Geometry: final body of the model. Coordinates: model frame, mm. Face numbers are marked on the shaded views. A direction names the side the tool comes from. Coordinates: 2 decimals unless noted, no trailing zeros. Order: outer loops, then holes, each group sorted by start corner. A loop starts at its lowest first (then second) coordinate and runs counter-clockwise, first axis right, second up. Notation, with made-up numbers: (40, -25) -> (86, -25) arc R24 cw to (86, -3) -> close; hole circle Ø7 at (85.5, 36). An arc over 180 degrees is marked (long way). Use one line per item in the form item = value.
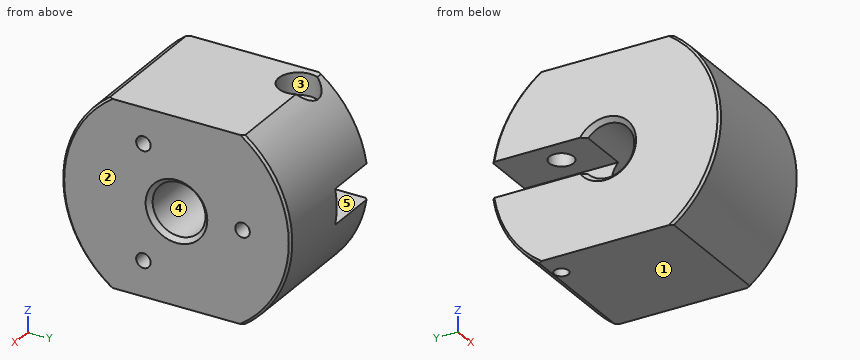
```python
from build123d import *

# Parameters (mm, degrees)
BOSS_EXTRUDE1_DEPTH                     = 30
CUT_EXTRUDE1_DEPTH                      = 12.5
SKETCH3_W                               = 30
SKETCH3_H                               = 6
HOLE1_D                                 = 5.08
HOLE1_DEPTH                             = 8.413530316
HOLE1_TIP                               = 1.466469684
SKETCH6_W                               = 1.621
SKETCH6_H                               = 17
CBORE_FOR_M5_HEX_HEAD_BOLT1_D           = 5.5118
CBORE_FOR_M5_HEX_HEAD_BOLT1_DEPTH       = 17
CBORE_FOR_M5_HEX_HEAD_BOLT1_CBORE_D     = 9
CBORE_FOR_M5_HEX_HEAD_BOLT1_CBORE_DEPTH = 5
CHAMFER1_SIZE                           = 0.5
CHAMFER2_SIZE                           = 1
CHAMFER3_SIZE                           = 0.379
M4_TAPPED_HOLE1_D                       = 3.3
M4_TAPPED_HOLE1_DEPTH                   = 8
M4_TAPPED_HOLE1_TIP                     = 0.991420021


with BuildPart() as part:
    # Sketch1 → Boss-Extrude1 (new body)
    with BuildSketch(Plane(origin=(0, 0, 0), x_dir=(0, 0, -1), z_dir=(1, 0, 0))):
        with BuildLine():
            Line((21, -15.329709717), (21, 15.329709717))
            ThreePointArc((21, 15.329709717), (0, 26), (-21, 15.329709717))
            Line((-21, 15.329709717), (-21, -15.329709717))
            ThreePointArc((-21, -15.329709717), (0, -26), (21, -15.329709717))
        make_face()
    extrude(amount=-BOSS_EXTRUDE1_DEPTH)

    # Sketch2 → Cut-Extrude1 (cut)
    with BuildSketch(Plane.ZY.offset(30)):
        with BuildLine():
            Line((-4, 25.690465157), (-4, 4.472135955))
            ThreePointArc((-4, 4.472135955), (0, 6), (4, 4.472135955))
            Line((4, 4.472135955), (4, 25.690465157))
            ThreePointArc((4, 25.690465157), (0, 26), (-4, 25.690465157))
        make_face()
    extrude(amount=-CUT_EXTRUDE1_DEPTH, mode=Mode.SUBTRACT)

    # Sketch3 → Cut-Revolve1 (revolve, cut)
    with BuildSketch(Plane.XY):
        with Locations((-15, 3)):
            Rectangle(SKETCH3_W, SKETCH3_H)
    revolve(axis=Axis((-30, 0, 0), (1, 0, 0)), mode=Mode.SUBTRACT)

    # Hole1
    with Locations(Plane.ZY.offset(17.5)):
        with Locations((0, 21.27272472)):
            Hole(HOLE1_D / 2, depth=HOLE1_DEPTH)
            with Locations((0, 0, -(HOLE1_DEPTH + HOLE1_TIP / 2))):  # 120° drill point
                Cone(0, HOLE1_D / 2, HOLE1_TIP, mode=Mode.SUBTRACT)

    # Sketch6 → M3 Clearance Hole1 (revolve, cut)
    with BuildSketch(Plane(origin=(-24, 13.5, -4), x_dir=(0, -1, 0), z_dir=(1, 0, 0))):
        with Locations((0.8105, 8.5)):
            Rectangle(SKETCH6_W, SKETCH6_H)
    revolve(axis=Axis((-24, 13.5, 2.35), (0, 0, -1)), mode=Mode.SUBTRACT)

    # CBORE for M5 Hex Head Bolt1
    with Locations(Plane.XY.offset(21)):
        with Locations((-24, 13.5)):
            CounterBoreHole(CBORE_FOR_M5_HEX_HEAD_BOLT1_D / 2, CBORE_FOR_M5_HEX_HEAD_BOLT1_CBORE_D / 2, CBORE_FOR_M5_HEX_HEAD_BOLT1_CBORE_DEPTH, depth=CBORE_FOR_M5_HEX_HEAD_BOLT1_DEPTH)

    # Chamfer1
    chamfer1_edges = [part.edges().sort_by_distance(p)[0] for p in [
        (-30, 22.201659548, -13.530939115),
        (-30, 22.201659548, 13.530939115),
        (-30, -26, 0),
        (0, 26, 0),
        (0, -26, 0),
    ]]
    chamfer(chamfer1_edges, length=CHAMFER1_SIZE)

    # Chamfer2
    chamfer2_edges = [part.edges().sort_by_distance(p)[0] for p in [
        (-30, -6, 0),
        (0, -6, 0),
    ]]
    chamfer(chamfer2_edges, length=CHAMFER2_SIZE)

    # Chamfer3
    chamfer3_edges = [part.edges().sort_by_distance(p)[0] for p in [
        (-24, 15.121, -4),
    ]]
    chamfer(chamfer3_edges, length=CHAMFER3_SIZE)

    # M4 Tapped Hole1
    with Locations(Plane(origin=(0, 0, 0), x_dir=(0, 0, -1), z_dir=(1, 0, 0))):
        with Locations((0, 15), (12.990381057, -7.5), (-12.990381057, -7.5), (0, 0)):
            Hole(M4_TAPPED_HOLE1_D / 2, depth=M4_TAPPED_HOLE1_DEPTH)
            with Locations((0, 0, -(M4_TAPPED_HOLE1_DEPTH + M4_TAPPED_HOLE1_TIP / 2))):  # 118° drill point
                Cone(0, M4_TAPPED_HOLE1_D / 2, M4_TAPPED_HOLE1_TIP, mode=Mode.SUBTRACT)


solid = part.part
```
1) Access query for the marked faces 4 and 5. Directions: +Z, -Z, +X, -X, +Y, -Y. A direction counts if a zero-diameter tool reaches every point of the face in a straight line with its end or side. Return the directions, or none.
Results found:
face_4 = +X, -X
face_5 = -X, +Y
2) Section C-C, the plane x = -24. Output: boundary loops of the cut face in (y, z).
Results found:
outline = (-15.33, -21) -> (11.88, -21) -> (11.88, -4.38) -> (11.5, -4) -> (4.47, -4) arc R6 cw (long way) to (4.47, 4) -> (10.74, 4) -> (10.74, 16) -> (9, 16) -> (9, 21) -> (-15.33, 21) arc R26 ccw to start; (15.12, -21) -> (15.33, -21) arc R26 ccw to (25.69, -4) -> (15.5, -4) -> (15.12, -4.38) -> close; (16.26, 4) -> (25.69, 4) arc R26 ccw to (18, 18.76) -> (18, 16) -> (16.26, 16) -> close
3) Pull-direction query (X, two-part tool) for the marked faces 1, 2 and 3; classes: released by +X, released by -X, zero draft, split by the parting line, or undercut.
Results found:
face_1 = zero draft
face_2 = released by +X
face_3 = undercut
4) Contact query for flat-ended pins moving along their axis: P1, Ø2, axis at x = -24.5, z = -12.5, coming from the -Y side; P2, Ø3, axis at y = -7.5, z = 12.99, coming from the +X side; P3, Ø10, axis at x = -25, y = 14.5, coming from the -Z side; P4, Ø4.5, axis at y = 21.27, z = 0, coming from the -X side. Output: stop coordinate, or through.
Results found:
P1 = -23.32
P2 = -8.09
P3 = -21
P4 = -8.92
5) Material intervals for probe 1 along Y at (x, z) = (-14.75, 0); probe 2 along Y at (x, z) = (-3, 0); probe 3 along Z at (x, y) = (-3, -7.5), sorted ascending. Write a range as from..to.
Results found:
probe_1 = -26..-6, 6..18.73, 23.81..26
probe_2 = -26..-6, 6..13.35, 16.65..26
probe_3 = -21..-14.64, -11.34..11.34, 14.64..21
6) Section A-A, the plane y = 0. Output: boundary loops of the cut face in (x, z), and give its area (3 significant figures).
Results found:
outline = (-30, -21) -> (0, -21) -> (0, -7) -> (-1, -6) -> (-29, -6) -> (-30, -7) -> close; (-30, 7) -> (-29, 6) -> (-1, 6) -> (0, 7) -> (0, 21) -> (-30, 21) -> close
area = 898 mm2
7) Section B-B, the plane x = -3. Output: boundary loops of the cut face in (y, z), and give its area (3 significant figures).
Results found:
outline = (-15.33, -21) -> (15.33, -21) arc R26 ccw to (15.33, 21) -> (-15.33, 21) arc R26 ccw to start; hole circle Ø3.3 at (-7.5, -12.99); hole circle Ø3.3 at (-7.5, 12.99); hole circle Ø12 at (0, 0); hole circle Ø3.3 at (15, 0)
area = 1,780 mm2
